```python
from build123d import *

# Parameters (mm, degrees)
SKETCH_W         = 60
SKETCH_H         = 25
PAD_DEPTH        = 7.25
HOLE_D           = 5
HOLE_DEPTH       = 25
HOLE_CBORE_D     = 6.2
HOLE_CBORE_DEPTH = 1.6
POCKET_DEPTH     = 4.5
POCKET001_DEPTH  = 60.001
FILLET_R         = 1.5


with BuildPart() as part:
    # Sketch → Pad (new body)
    with BuildSketch(Plane.XY):
        with Locations((0, 2.5)):
            Rectangle(SKETCH_W, SKETCH_H)
    extrude(amount=PAD_DEPTH)

    # Hole
    with Locations(Plane(origin=(0, 0, 0), x_dir=(1, 0, 0), z_dir=(0, 0, -1))):
        with Locations((-12.5, 0), (12.5, 0)):
            CounterBoreHole(HOLE_D / 2, HOLE_CBORE_D / 2, HOLE_CBORE_DEPTH, depth=HOLE_DEPTH)

    # Sketch002 (on Face5 of Hole) → Pocket (cut)
    with BuildSketch(Plane.XY.offset(7.25)):
        Polygon((-10.190599, 4), (-14.809401, 4), (-17.118802, 0), (-14.809401, -4), (-10.190599, -4), (-7.881198, 0), align=None)
        Polygon((10.190599, 4), (7.881198, 0), (10.190599, -4), (14.809401, -4), (17.118802, 0), (14.809401, 4), align=None)
    extrude(amount=-POCKET_DEPTH, mode=Mode.SUBTRACT)

    # Sketch003 (on Face2 of Pocket) → Pocket001 (cut, through all)
    with BuildSketch(Plane(origin=(-30, 0, 0), x_dir=(0, -1, 0), z_dir=(-1, 0, 0))):
        Polygon((-7.5, 4.116025), (-9, 4.982051), (-10.5, 4.116025), (-10.5, 2.383975), (-9, 1.517949), (-7.5, 2.383975), align=None)
    extrude(amount=-POCKET001_DEPTH, mode=Mode.SUBTRACT)

    # Fillet
    fillet_edges = [part.edges().sort_by_distance(p)[0] for p in [
        (-30, -10, 3.625),
        (-30, 2.5, 7.25),
        (0, 15, 7.25),
        (0, -10, 7.25),
        (-30, 15, 3.625),
        (30, 2.5, 7.25),
        (30, -10, 3.625),
        (30, 15, 3.625),
    ]]
    fillet(fillet_edges, radius=FILLET_R)


solid = part.part
```
Source: CAD feature listing. Evaluate the final solid. Frame: model axes, mm. A direction names the side the tool comes from. Coordinates: 2 decimals unless noted, no trailing zeros. Write each loop counter-clockwise with the first axis right and the second up, starting at its lowest first coordinate (ties: lowest second). Pieces come first, ordered by that corner, then holes. Notation, with made-up numbers: M 59,40 L 80,40 A23 ccw 80,67 Z; hole C -26.5,63 d9. An arc over 180 degrees is marked long. Answer as a JSON object with one key per item and string values.
1. Cut plane B-B on x = 1. Output: boundary loops of the cut face in (y, z).
Evaluation:
{"outline": "M -10,0 L 15,0 L 15,5.75 A1.5 ccw 13.5,7.25 L -8.5,7.25 A1.5 ccw -10,5.75 Z; hole M 7.5,2.38 L 9,1.52 L 10.5,2.38 L 10.5,4.12 L 9,4.98 L 7.5,4.12 Z"}
2. Ray query, L1, parallel to Y at x = 26, z = 3; L2, parallel to Y at x = -12.5, z = 1.25; L3, parallel to X at y = -1.75, z = 1.75. Return the intervals inside material, ascending.
Evaluation:
{"L1": "-10 to 7.5, 10.5 to 15", "L2": "-10 to -3.1, 3.1 to 15", "L3": "-30 to -14.29, -10.71 to 10.71, 14.29 to 30"}
3. Access query for faces 4 (the flat face through (10, -1, 1.6)), 5 (the flat face through (0, 15, 3)), 6 (the flat face through (0, 3, 0)), 7 (the flat face through (-10.5, 1.8, 2.75)), 8 (the flat face through (-0.42, 9.76, 1.957)). Directions: +Z, -Z, +X, -X, +Y, -Y. A direction counts if a zero-diameter tool reaches every point of the face in a straight line with its end or side. Return the directions, or none.
Evaluation:
{"face 4": "-Z", "face 5": "+Z, -Z, +X, -X, +Y", "face 6": "-Z, +X, -X, +Y, -Y", "face 7": "+Z", "face 8": "+X, -X"}
4. Cut plane A-A on x = 12.5. Output: boundary loops of the cut face in (y, z).
Evaluation:
{"outline": "M -10,0 L -3.1,0 L -3.1,1.6 L -2.5,1.6 L -2.5,2.75 L -4,2.75 L -4,7.25 L -8.5,7.25 A1.5 ccw -10,5.75 Z; M 2.5,1.6 L 3.1,1.6 L 3.1,0 L 15,0 L 15,5.75 A1.5 ccw 13.5,7.25 L 4,7.25 L 4,2.75 L 2.5,2.75 Z; hole M 7.5,2.38 L 9,1.52 L 10.5,2.38 L 10.5,4.12 L 9,4.98 L 7.5,4.12 Z"}
5. Cut plane D-D on x = -14. Output: boundary loops of the cut face in (y, z), plus the area to 3 significant figures.
Evaluation:
{"outline": "M -10,0 L -2.71,0 L -2.71,1.6 L -2,1.6 L -2,2.75 L -4,2.75 L -4,7.25 L -8.5,7.25 A1.5 ccw -10,5.75 Z; M 2,1.6 L 2.71,1.6 L 2.71,0 L 15,0 L 15,5.75 A1.5 ccw 13.5,7.25 L 4,7.25 L 4,2.75 L 2,2.75 Z; hole M 7.5,2.38 L 9,1.52 L 10.5,2.38 L 10.5,4.12 L 9,4.98 L 7.5,4.12 Z", "area": "123 mm^2"}
6. Cut plane C-C on y = 1.25. State how many separate pieces and enclosed holes the cut face has, plus the area to 3 significant figures.
Evaluation:
{"separate pieces": "3", "enclosed holes": "0", "area": "336 mm^2"}
7. Contact query for flat-ended pins moving along their axis: P1, Ø5.5, axis at x = 12.5, y = 0, coming from the +Z side; P2, Ø6.5, axis at x = 12.5, y = 0, coming from the -Z side; P3, Ø1.9, axis at x = 13, y = -1.5, coming from the -Z side. Output: stop coordinate, or through.
Evaluation:
{"P1": "z = 2.75", "P2": "z = 0", "P3": "z = 1.6"}
8. Draft query along Y for faces 1 (the flat face through (-30, 2, 3)), 2 (the cylindrical face through (29.55, 14.57, 2.92)), 3 (the flat face through (12, -4, 5)). Return one class per face: released by +Y, released by -Y, zero draft, split by the parting line, or undercut.
Evaluation:
{"face 1": "zero draft", "face 2": "released by +Y", "face 3": "undercut"}
